Could you check a few things on this model? Use its own coordinates, in mm. Coordinates: 2 decimals unless noted, no trailing zeros. Order: outer loops, then holes, each group sorted by start corner. A loop starts at its lowest first (then second) coordinate and runs counter-clockwise, first axis right, second up. Notation, with made-up numbers: (60, 17.25) - (67, 17.25) arc R7 ccw to (67, 21.25) - close; hole circle Ø11 at (60.5, -10). An arc over 180 degrees is marked (long way). Answer as a JSON object with one key per item and string values. Group by question number.
(1) Imagine slicing it at A-A, the plane x = 0. Write out the boundary of the cut face in (y, z), and give its area (3 significant figures).
(2) Imagine slicing it at B-B, the plane x = -38.3. Write out the boundary of the cut face in (y, z).
(3) Please list where these lines run through material, in increasing order: probe 1 along Y at (x, z) = (0, 2.9); probe 2 along Y at (x, z) = (2.5, 0.5); probe 3 along X at (y, z) = (48, 1.15).
(4) Imagine slicing it at C-C, the plane x = 26. Write out the boundary of the cut face in (y, z), and give its area (3 significant figures).
(5) Imagine slicing it at D-D, the plane z = 4.2. Give the number of separate pieces and of enclosed holes in the cut face, and give its area (3 significant figures).
(6) Will this pin go through, and if not, where does the flat tip stop? P1, Ø3, axis at x = 38.3, y = 30.35, coming from the +Z side.
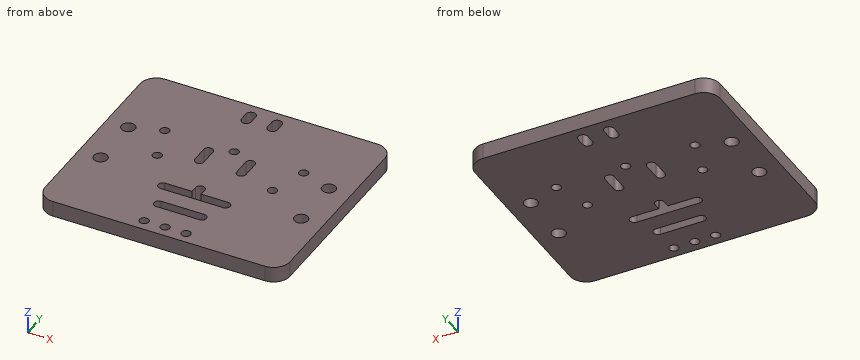
from build123d import *

# Parameters (mm, degrees)
MODEL_R                    = 1.75
BASE_DEPTH                 = 6
F_5_2_5_2_DIAMETER_HOLE1_D = 5.2


with BuildPart() as part:
    # Model → Base (new body)
    with BuildSketch(Plane.XY):
        with BuildLine():
            Line((46.75, 74.75), (46.75, 6.25))
            ThreePointArc((46.75, 6.25), (44.919417382, 1.830582618), (40.5, 0))
            Line((40.5, 0), (-40.5, 0))
            ThreePointArc((-40.5, 0), (-44.919417382, 1.830582618), (-46.75, 6.25))
            Line((-46.75, 6.25), (-46.75, 74.75))
            ThreePointArc((-46.75, 74.75), (-44.919417382, 79.169417382), (-40.5, 81))
            Line((-40.5, 81), (40.5, 81))
            ThreePointArc((40.5, 81), (44.919417382, 79.169417382), (46.75, 74.75))
        make_face()
        with Locations((0, 4.5)):
            Circle(MODEL_R, mode=Mode.SUBTRACT)
        with Locations((8, 4.5)):
            Circle(MODEL_R, mode=Mode.SUBTRACT)
        with Locations((-8, 4.5)):
            Circle(MODEL_R, mode=Mode.SUBTRACT)
        with Locations((0, 54.4)):
            Circle(MODEL_R, mode=Mode.SUBTRACT)
        with Locations((26.5, 54.4)):
            Circle(MODEL_R, mode=Mode.SUBTRACT)
        with Locations((22, 40.4)):
            Circle(MODEL_R, mode=Mode.SUBTRACT)
        with Locations((-22, 40.4)):
            Circle(MODEL_R, mode=Mode.SUBTRACT)
        with Locations((-26.5, 54.4)):
            Circle(MODEL_R, mode=Mode.SUBTRACT)
        with BuildLine():
            Line((-3.1, 75.8), (-3.1, 72.6))
            ThreePointArc((-3.1, 72.6), (-5, 70.7), (-6.9, 72.6))
            Line((-6.9, 72.6), (-6.9, 75.8))
            ThreePointArc((-6.9, 75.8), (-5, 77.7), (-3.1, 75.8))
        make_face(mode=Mode.SUBTRACT)
        with BuildLine():
            Line((-9.75, 50.9), (-9.75, 44.4))
            ThreePointArc((-9.75, 44.4), (-8, 42.65), (-6.25, 44.4))
            Line((-6.25, 44.4), (-6.25, 50.9))
            ThreePointArc((-6.25, 50.9), (-8, 52.65), (-9.75, 50.9))
        make_face(mode=Mode.SUBTRACT)
        with BuildLine():
            Line((3.1, 72.6), (3.1, 75.8))
            ThreePointArc((3.1, 75.8), (5, 77.7), (6.9, 75.8))
            Line((6.9, 75.8), (6.9, 72.6))
            ThreePointArc((6.9, 72.6), (5, 70.7), (3.1, 72.6))
        make_face(mode=Mode.SUBTRACT)
        with BuildLine():
            Line((8.25, 17.25), (-8.25, 17.25))
            ThreePointArc((-8.25, 17.25), (-10, 15.5), (-8.25, 13.75))
            Line((-8.25, 13.75), (8.25, 13.75))
            ThreePointArc((8.25, 13.75), (10, 15.5), (8.25, 17.25))
        make_face(mode=Mode.SUBTRACT)
        with BuildLine():
            Line((9.75, 44.4), (9.75, 50.9))
            ThreePointArc((9.75, 50.9), (8, 52.65), (6.25, 50.9))
            Line((6.25, 50.9), (6.25, 44.4))
            ThreePointArc((6.25, 44.4), (8, 42.65), (9.75, 44.4))
        make_face(mode=Mode.SUBTRACT)
        with BuildLine():
            Line((-1.75, 29.85), (-1.75, 27.25))
            Line((-1.75, 27.25), (-12, 27.25))
            ThreePointArc((-12, 27.25), (-13.75, 25.5), (-12, 23.75))
            Line((-12, 23.75), (12, 23.75))
            ThreePointArc((12, 23.75), (13.75, 25.5), (12, 27.25))
            Line((12, 27.25), (1.75, 27.25))
            Line((1.75, 27.25), (1.75, 29.85))
            ThreePointArc((1.75, 29.85), (0, 31.6), (-1.75, 29.85))
        make_face(mode=Mode.SUBTRACT)
    extrude(amount=BASE_DEPTH)

    # Ø5.2 (5.2) Diameter Hole1 (through all)
    with Locations(Plane.XY.offset(6)):
        with Locations((-38.3, 50.35), (-38.3, 30.35), (38.3, 30.35), (38.3, 50.35)):
            Hole(F_5_2_5_2_DIAMETER_HOLE1_D / 2)


solid = part.part
Result set:
{
 "1": {"outline": "(0, 0) - (2.75, 0) - (2.75, 6) - (0, 6) - close; (6.25, 0) - (13.75, 0) - (13.75, 6) - (6.25, 6) - close; (17.25, 0) - (23.75, 0) - (23.75, 6) - (17.25, 6) - close; (31.6, 0) - (52.65, 0) - (52.65, 6) - (31.6, 6) - close; (56.15, 0) - (81, 0) - (81, 6) - (56.15, 6) - close", "area": "376 mm^2"},
 "2": {"outline": "(0, 0) - (27.75, 0) - (27.75, 6) - (0, 6) - close; (32.95, 0) - (47.75, 0) - (47.75, 6) - (32.95, 6) - close; (52.95, 0) - (81, 0) - (81, 6) - (52.95, 6) - close"},
 "3": {"probe 1": "y = 0 to 2.75, 6.25 to 13.75, 17.25 to 23.75, 31.6 to 52.65, 56.15 to 81", "probe 2": "y = 0 to 13.75, 17.25 to 23.75, 27.25 to 81", "probe 3": "x = -46.75 to -39.41, -37.19 to -9.75, -6.25 to 6.25, 9.75 to 37.19, 39.41 to 46.75"},
 "4": {"outline": "(0, 0) - (52.72, 0) - (52.72, 6) - (0, 6) - close; (56.08, 0) - (81, 0) - (81, 6) - (56.08, 6) - close", "area": "466 mm^2"},
 "5": {"separate pieces": "1", "enclosed holes": "18", "area": "7,090 mm^2"},
 "6": {"P1": "passes through"}
}
